CAD build for the part. Positions are in the model's coordinates, mm. A direction names the side the tool comes from. Round coordinates to 2 decimals unless told otherwise and drop trailing zeros. Write each loop counter-clockwise with the first axis right and the second up, starting at its lowest first coordinate (ties: lowest second). Pieces come first, ordered by that corner, then holes. Notation, with made-up numbers: (5.25, -7) - (13.25, -7) arc R10 ccw to (13.25, 4) - close; hole circle Ø7 at (-16, 44.25). An arc over 180 degrees is marked (long way). Use one line per item in the form item = value. Start each with the question number.
Item 1: Tool access for faces 1 (the flat face through (51.275, -1, 3)), 2 (the cylindrical face through (-26.826, -34.984, -2.218)), 3 (the cylindrical face through (-0.16, 33.79, 13.15)): list every direction of +Z, -Z, +X, -X, +Y, -Y with a clear straight run to the whole face (end or side of a thin tool).
Item 2: Band-saw the part on A-A, the plane x = 0. List the corners of the cut face in (y, z).
Item 3: Pin check, flat tips, straight feed: pin 1 (12 mm diameter, centred on x = 4, y = 27, fed in from -Z); pin 2 (4 mm diameter, centred on x = 15, y = -27, fed in from -Z); pin 3 (8 mm diameter, centred on x = 27, z = -5.5, fed in from -Y). Stop position of each tip, or through.
Item 4: Band-saw the part on B-B, the plane y = 32.55. List the corners of the cut face in (x, z) (3 decimals), and give its area (3 significant figures).
Item 5: Band-saw the part on C-C, the plane z = 7.75. List the corners of the cut face in (x, y), and give its area (3 significant figures).
Item 6: Band-saw the part on D-D, the plane x = 15. List the corners of the cut face in (y, z).
Item 7: Drill centre lines: L1, parallel to Z at x = -46, y = 12; L2, parallel to Z at x = 1.5, y = 30.5; L3, parallel to Y at x = -16, z = -4. Where is each one in solid material? Low to high.
Item 8: Pull direction X, two halves, no side cores. Call faces 4 (the flat face through (-32, -32, -4.5)), 5 (the flat face through (-51.275, -1, 3)), 6 (the flat face through (2, 33, 10.44)), 7 (the cylindrical face through (18.996, -32.374, -2.218)): +X half, -X half, draft (parallel to the pull), parting line (faces both ways), or undercut.
from build123d import *

# Parameters (mm, degrees)
SKETCH1_W           = 102.55
SKETCH1_H           = 77.1
BOSS_EXTRUDE1_DEPTH = 5.94
SKETCH2_R           = 4
BOSS_EXTRUDE2_DEPTH = 4.5
SKETCH3_R           = 1.25
BOSS_EXTRUDE3_DEPTH = 5.5
SKETCH5_R           = 4
BOSS_EXTRUDE4_DEPTH = 4.5
SKETCH6_R           = 1.25
BOSS_EXTRUDE5_DEPTH = 5.5


with BuildPart() as part:
    # Sketch1 → Boss-Extrude1 (new body)
    with BuildSketch(Plane.XY):
        Rectangle(SKETCH1_W, SKETCH1_H)
    extrude(amount=BOSS_EXTRUDE1_DEPTH)

    # Sketch2 → Boss-Extrude2 (add)
    with BuildSketch(Plane(origin=(0, 0, 0), x_dir=(-1, 0, 0), z_dir=(0, 0, -1))):
        with Locations((-30, -32.55)):
            Circle(SKETCH2_R)
        with Locations((-15, -32.55)):
            Circle(SKETCH2_R)
        with Locations((0, -32.55)):
            Circle(SKETCH2_R)
        with Locations((15, -32.55)):
            Circle(SKETCH2_R)
        with Locations((30, -32.55)):
            Circle(SKETCH2_R)
    extrude(amount=BOSS_EXTRUDE2_DEPTH)

    # Sketch3 → Boss-Extrude3 (add)
    with BuildSketch(Plane(origin=(0, 0, -4.5), x_dir=(-1, 0, 0), z_dir=(0, 0, -1))):
        with Locations((-30, -32.55)):
            Circle(SKETCH3_R)
        with Locations((-15, -32.55)):
            Circle(SKETCH3_R)
        with Locations((0, -32.55)):
            Circle(SKETCH3_R)
        with Locations((15, -32.55)):
            Circle(SKETCH3_R)
        with Locations((30, -32.55)):
            Circle(SKETCH3_R)
    extrude(amount=BOSS_EXTRUDE3_DEPTH)

    # Sketch5 → Boss-Extrude4 (add)
    with BuildSketch(Plane.XY.offset(5.94)):
        with Locations((0, 32.55)):
            Circle(SKETCH5_R)
    extrude(amount=BOSS_EXTRUDE4_DEPTH)

    # Sketch6 → Boss-Extrude5 (add)
    with BuildSketch(Plane.XY.offset(10.44)):
        with Locations((0, 32.55)):
            Circle(SKETCH6_R)
    extrude(amount=BOSS_EXTRUDE5_DEPTH)


solid = part.part
Determined:
q1.face_1 = +Z, -Z, +X, +Y, -Y
q1.face_2 = -Z
q1.face_3 = +Z
q2.outline = (-38.55, 0) - (-36.55, 0) - (-36.55, -4.5) - (-33.8, -4.5) - (-33.8, -10) - (-31.3, -10) - (-31.3, -4.5) - (-28.55, -4.5) - (-28.55, 0) - (38.55, 0) - (38.55, 5.94) - (36.55, 5.94) - (36.55, 10.44) - (33.8, 10.44) - (33.8, 15.94) - (31.3, 15.94) - (31.3, 10.44) - (28.55, 10.44) - (28.55, 5.94) - (-38.55, 5.94) - close
q3.pin_1 = 0
q3.pin_2 = -4.5
q3.pin_3 = -36.55
q4.outline = (-51.275, 0) - (51.275, 0) - (51.275, 5.94) - (4, 5.94) - (4, 10.44) - (1.25, 10.44) - (1.25, 15.94) - (-1.25, 15.94) - (-1.25, 10.44) - (-4, 10.44) - (-4, 5.94) - (-51.275, 5.94) - close
q4.area = 659 mm²
q5.outline = circle Ø8 at (0, 32.55)
q5.area = 50.3 mm²
q6.outline = (-38.55, 0) - (-36.55, 0) - (-36.55, -4.5) - (-33.8, -4.5) - (-33.8, -10) - (-31.3, -10) - (-31.3, -4.5) - (-28.55, -4.5) - (-28.55, 0) - (38.55, 0) - (38.55, 5.94) - (-38.55, 5.94) - close
q7.L1 = 0 to 5.94
q7.L2 = 0 to 10.44
q7.L3 = -36.42 to -28.68
q8.face_4 = undercut
q8.face_5 = -X half
q8.face_6 = draft
q8.face_7 = undercut
